from build123d import *

# Parameters (mm, degrees)
SKETCH_1_R          = 2.45875
EXTRUDE_640_DEPTH   = 5.7
SKETCH_2_OUTSIDE_W  = 51.738
SKETCH_2_OUTSIDE_H  = 53.286
SKETCH_2_OUTSIDE_R  = 5
CUT_EXTRUDE_1_DEPTH = 10.530127666
CUT_EXTRUDE_1_DRAFT = -60
CHAMFER_1_SIZE      = 0.91625
SKETCH_3_OUTSIDE_W  = 51.738
SKETCH_3_OUTSIDE_H  = 53.286
SKETCH_3_OUTSIDE_R  = 5
CUT_EXTRUDE_2_DEPTH = 10.530127666
CUT_EXTRUDE_2_DRAFT = -60
SKETCH_4_R          = 8.9
SKETCH_4_R_2        = 4.45
CUT_EXTRUDE_3_DEPTH = 0.5


with BuildPart() as part:
    # 草图1 → Extrude 640 (new body)
    with BuildSketch(Plane.XY):
        Polygon((0, 5.773502692), (-5, 2.886751346), (-5, -2.886751346), (0, -5.773502692), (5, -2.886751346), (5, 2.886751346), align=None)
        Circle(SKETCH_1_R, mode=Mode.SUBTRACT)
    extrude(amount=EXTRUDE_640_DEPTH)


with BuildPart() as cut_extrude_1_tool:
    # 草图2 outside → 切除-拉伸1 (with draft: the straight prism first)
    with BuildSketch(Plane(origin=(0, 0, 0), x_dir=(-1, 0, 0), z_dir=(0, 0, -1))):
        Rectangle(SKETCH_2_OUTSIDE_W, SKETCH_2_OUTSIDE_H)
        Circle(SKETCH_2_OUTSIDE_R, mode=Mode.SUBTRACT)
    extrude(amount=-CUT_EXTRUDE_1_DEPTH)
    # 切除-拉伸1: the draft: its side faces are tilted about the plane it starts from
    cut_extrude_1_sides = [cut_extrude_1_tool.faces().sort_by_distance(p)[0] for p in [
        (0, -26.643, 5.265063833),
        (-25.869, 0, 5.265063833),
        (0, 26.643, 5.265063833),
        (25.869, 0, 5.265063833),
        (5, 0, 5.265063833),
    ]]
    draft(cut_extrude_1_sides, Plane(origin=(0, 0, 0), x_dir=(-1, 0, 0), z_dir=(0, 0, -1)), CUT_EXTRUDE_1_DRAFT)


with BuildPart() as part_1:
    add(part.part)

    # 切除-拉伸1: cut by cut_extrude_1_tool
    add(cut_extrude_1_tool.part, mode=Mode.SUBTRACT)

    # 倒角1
    chamfer_1_edges = [part_1.edges().sort_by_distance(p)[0] for p in [
        (-2.45875, 0, 0),
        (-2.45875, 0, 5.7),
    ]]
    chamfer(chamfer_1_edges, length=CHAMFER_1_SIZE)


with BuildPart() as cut_extrude_2_tool:
    # 草图3 outside → 切除-拉伸2 (with draft: the straight prism first)
    with BuildSketch(Plane.XY.offset(5.7)):
        Rectangle(SKETCH_3_OUTSIDE_W, SKETCH_3_OUTSIDE_H)
        Circle(SKETCH_3_OUTSIDE_R, mode=Mode.SUBTRACT)
    extrude(amount=-CUT_EXTRUDE_2_DEPTH)
    # 切除-拉伸2: the draft: its side faces are tilted about the plane it starts from
    cut_extrude_2_sides = [cut_extrude_2_tool.faces().sort_by_distance(p)[0] for p in [
        (0, -26.643, 0.434936167),
        (25.869, 0, 0.434936167),
        (0, 26.643, 0.434936167),
        (-25.869, 0, 0.434936167),
        (-5, 0, 0.434936167),
    ]]
    draft(cut_extrude_2_sides, Plane.XY.offset(5.7), CUT_EXTRUDE_2_DRAFT)


with BuildPart() as part_2:
    add(part_1.part)

    # 切除-拉伸2: cut by cut_extrude_2_tool
    add(cut_extrude_2_tool.part, mode=Mode.SUBTRACT)

    # 草图4 → 切除-拉伸3 (cut)
    with BuildSketch(Plane.XY.offset(5.7)):
        Circle(SKETCH_4_R)
        Circle(SKETCH_4_R_2, mode=Mode.SUBTRACT)
    extrude(amount=-CUT_EXTRUDE_3_DEPTH, mode=Mode.SUBTRACT)


solid = part_2.part
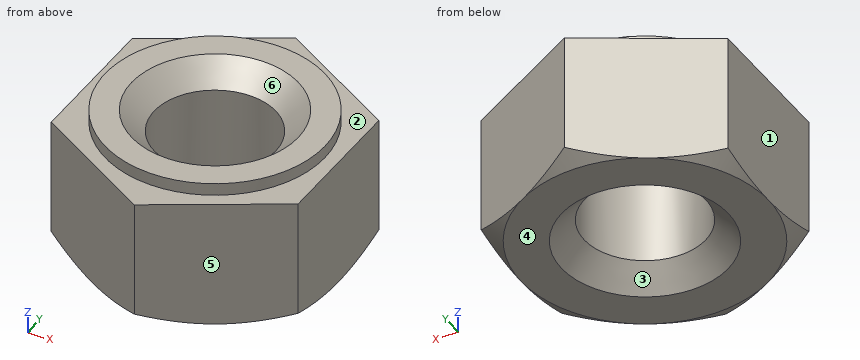
The listing builds one solid part. Answer for the finished solid, in the listing's coordinates (mm). Face numbers are marked on the shaded views. A direction names the side the tool comes from. Round coordinates to 2 decimals unless told otherwise and drop trailing zeros. Order: outer loops, then holes, each group sorted by start corner. A loop starts at its lowest first (then second) coordinate and runs counter-clockwise, first axis right, second up. Notation, with made-up numbers: (29.5, 34) -> (47.5, 34) arc R17 ccw to (47.5, 66) -> close; hole circle Ø3 at (0, 3.5). An arc over 180 degrees is marked (long way). Put each result on its own line as item: value.
Q1. Determine the mould class of the marked faces 3, 4, 5 and 6 for opening direction X: pulls with the +X half, pulls with the -X half, needs draft (parallel to the pull), parting line crosses it, or undercut.
Results list:
face 3: undercut
face 4: needs draft
face 5: pulls with the +X half
face 6: undercut
Q2. Each of these flat-tipped pins is pushed along its axis until it touches: P1, Ø1, axis at x = -2, y = -2, coming from the +Z side; P2, Ø3, axis at y = 4.5, z = 2.5, coming from the -X side. Where does it stop, or does it pass through?
Results list:
P1: z = 5.65
P2: x = -4.8
Q3. Section A-A, the plane z = 2.2 is taken. Write down the section's boundary in (x, y), and give its area (3 significant figures).
Results list:
outline: (-5, -2.89) -> (0, -5.77) -> (5, -2.89) -> (5, 2.89) -> (0, 5.77) -> (-5, 2.89) -> close; hole circle Ø4.92 at (0, 0)
area: 67.6 mm^2
Q4. Which of the six approach directions +Z, -Z, +X, -X, +Y, -Y give full straight-line access (tool end or side, diameter ignored) to the marked faces 1 and 2?
Results list:
face 1: +Z, -Z, -X, +Y, -Y
face 2: +Z
Q5. Consider line 1 along Y through (x, z) = (-2.5, 2.8); line 2 along X through (y, z) = (1.5, 2.1); line 3 along Z through (x, y) = (-1.5, 4.5). Determine where each line is inside the solid, lowest interval first.
Results list:
line 1: -4.33 to 4.33
line 2: -5 to -1.95, 1.95 to 5
line 3: 0 to 5.2
